The model under review builds one solid part; all positions refer to its coordinate system, in mm. A direction names the side the tool comes from. Coordinates: 2 decimals unless noted, no trailing zeros. Order: outer loops, then holes, each group sorted by start corner. A loop starts at its lowest first (then second) coordinate and runs counter-clockwise, first axis right, second up. Notation, with made-up numbers: (-25.75, 35.5) -> (-10.75, 35.5) arc R17 cw to (-10.75, 47.5) -> close; hole circle Ø10 at (62.25, 68). An arc over 180 degrees is marked (long way). Put each result on its own line as item: value.
from build123d import *

# Parameters (mm, degrees)
BOSS_EXTRUDE1_DEPTH = 20
BOSS_EXTRUDE2_START = 10
BOSS_EXTRUDE2_DEPTH = 10
BOSS_EXTRUDE3_START = 50
BOSS_EXTRUDE3_DEPTH = 50
CHAMFER3_SIZE       = 6
SKETCH3_R           = 6
CUT_EXTRUDE1_DEPTH  = 50


with BuildPart() as part:
    # Sketch1 → Boss-Extrude1 (new body)
    with BuildSketch(Plane.XY):
        with BuildLine():
            ThreePointArc((13.076696831, 5), (0, 14), (-13.076696831, 5))
            Line((-13.076696831, 5), (13.076696831, 5))
        make_face()
        with BuildLine():
            Line((13.076696831, 5), (-13.076696831, 5))
            ThreePointArc((-13.076696831, 5), (-2.542267135, -13.767239295), (14, 0))
            ThreePointArc((14, 0), (13.767239295, 2.542267135), (13.076696831, 5))
        make_face()
        with BuildLine():
            ThreePointArc((19.364916731, 5), (0, 20), (-19.364916731, 5))
            Line((-19.364916731, 5), (-13.076696831, 5))
            ThreePointArc((-13.076696831, 5), (0, 14), (13.076696831, 5))
            Line((13.076696831, 5), (19.364916731, 5))
        make_face()
        with BuildLine():
            Line((-13.076696831, 5), (-19.364916731, 5))
            ThreePointArc((-19.364916731, 5), (-2.52008585, -19.840593925), (20, 0))
            ThreePointArc((20, 0), (19.840593925, 2.52008585), (19.364916731, 5))
            Line((19.364916731, 5), (13.076696831, 5))
            ThreePointArc((13.076696831, 5), (13.767239295, 2.542267135), (14, 0))
            ThreePointArc((14, 0), (-2.542267135, -13.767239295), (-13.076696831, 5))
        make_face()
    extrude(amount=-BOSS_EXTRUDE1_DEPTH)

    # Sketch1_4 → Boss-Extrude2 (add)
    with BuildSketch(Plane.XY.offset(BOSS_EXTRUDE2_START)):
        with BuildLine():
            Line((-13.076696831, 5), (-19.364916731, 5))
            ThreePointArc((-19.364916731, 5), (-2.52008585, -19.840593925), (20, 0))
            ThreePointArc((20, 0), (19.840593925, 2.52008585), (19.364916731, 5))
            Line((19.364916731, 5), (13.076696831, 5))
            ThreePointArc((13.076696831, 5), (13.767239295, 2.542267135), (14, 0))
            ThreePointArc((14, 0), (-2.542267135, -13.767239295), (-13.076696831, 5))
        make_face()
    extrude(amount=-BOSS_EXTRUDE2_DEPTH)

    # Sketch1_5 → Boss-Extrude3 (add)
    with BuildSketch(Plane.XY.offset(BOSS_EXTRUDE3_START)):
        with BuildLine():
            Line((13.076696831, 5), (-13.076696831, 5))
            ThreePointArc((-13.076696831, 5), (-2.542267135, -13.767239295), (14, 0))
            ThreePointArc((14, 0), (13.767239295, 2.542267135), (13.076696831, 5))
        make_face()
    extrude(amount=-BOSS_EXTRUDE3_DEPTH)

    # Chamfer3
    chamfer3_edges = [part.edges().sort_by_distance(p)[0] for p in [
        (-2.542267135, -13.767239295, 50),
    ]]
    chamfer(chamfer3_edges, length=CHAMFER3_SIZE)

    # Sketch3 → Cut-Extrude1 (cut)
    with BuildSketch(Plane(origin=(0, 5, 0), x_dir=(1, 0, 0), z_dir=(0, 1, 0))):
        with Locations(Location((0, -20, 0), (0, 0, 270))):
            Circle(SKETCH3_R)
    extrude(amount=-CUT_EXTRUDE1_DEPTH, mode=Mode.SUBTRACT)


solid = part.part
Item 1: For line 1 (Z direction, x = 0, y = -5); line 2 (Z direction, x = -7, y = -12.5); line 3 (X direction, y = 1, z = 17), list the stretches that pass through material, from the lowest coordinate up. Write a range as from..to.
Answers below:
line 1: -20..14, 26..50
line 2: -20..10
line 3: -13.96..-5.2, 5.2..13.96
Item 2: Mouldability with a two-part tool opening along Z and no side actions: class faces 1 (the flat face through (3, -14, 10)), 2 (the cylindrical face through (-2.3, -4.37, 25.54)), 3 (the flat face through (-4, 5, 25)) as +Z half, -Z half, draft (parallel to the pull), parting line (faces both ways), or undercut.
Answers below:
face 1: +Z half
face 2: undercut
face 3: draft
Item 3: Consider section D-D on x = -17. Write out the cut boundary in (y, z), and give its area (3 significant figures).
Answers below:
outline: (-10.54, -20) -> (10.54, -20) -> (10.54, 0) -> (5, 0) -> (5, 10) -> (-10.54, 10) -> close
area: 577 mm^2
Item 4: For pin 1 Ø12 at (y, z) = (-8, 28) entering from -X; pin 2 Ø8 at (x, z) = (13, -5) entering from +Y; pin 3 Ø12 at (x, z) = (-6, 28.5) entering from +Y; pin 4 Ø16.5 at (x, y) = (-2.5, 11.5) entering from +Z, all flat-tipped, find the tip position at first contact; note any pin that passes through.
Answers below:
pin 1: x = -13.86
pin 2: y = 17.86
pin 3: y = 5
pin 4: z = 50
Item 5: Consider section C-C on y = 14.5. Write out the cut boundary in (x, z), and give its area (3 significant figures).
Answers below:
outline: (-13.77, -20) -> (13.77, -20) -> (13.77, 0) -> (-13.77, 0) -> close
area: 551 mm^2
Item 6: Consider section A-A on x = 0. Write out the cut boundary in (y, z).
Answers below:
outline: (-20, -20) -> (20, -20) -> (20, 0) -> (5, 0) -> (5, 14) -> (-14, 14) -> (-14, 10) -> (-20, 10) -> close; (-14, 26) -> (5, 26) -> (5, 50) -> (-8, 50) -> (-14, 44) -> close
Item 7: Consider section B-B on z = 20. Write out the cut boundary in (x, y), and give its area (3 significant figures).
Answers below:
outline: (-13.08, 5) arc R14 ccw to (-6, -12.65) -> (-6, 5) -> close; (6, -12.65) arc R14 ccw to (13.08, 5) -> (6, 5) -> close
area: 222 mm^2
Item 8: For faces 4 (the flat face through (0, 11, 0)), 5 (the flat face through (0, 0, -20)), list the 3-axis set-ups (+Z, -Z, +X, -X, +Y, -Y) from which the entire face can be reached by the end or side of a thin tool; tool diameter is ignored.
Answers below:
face 4: +Z, +X, -X, +Y
face 5: -Z, +X, -X, +Y, -Y
